The model under review builds one solid part; all positions refer to its coordinate system, in mm. Coordinates: 2 decimals unless noted, no trailing zeros. Loops run counter-clockwise (first coordinate to the right, second up) from the corner with the lowest first, then second, coordinate; pieces in that order, holes last. Notation, with made-up numbers: M -35,-4 L -9,-4 A37 cw -9,34 Z; hole C -6.5,87 d3. An arc over 180 degrees is marked long. Use CSV: the item, a comma, the result in double quotes. Start each with the question number.
1. Add section A-A, the plane z = 119.5. Write out the cut boundary in (x, y).
2. Clearance check with flat-ended pins moving along their axes: P1, Ø1, axis at x = 230, y = 199.5, coming from the +Z side; P2, Ø0.6, axis at x = 237.5, y = 199.5, coming from the -Z side; P3, Ø1, axis at x = 233, y = 181.5, coming from the +Z side; P4, Ø2, axis at x = 232.5, z = 51.5, coming from the +Y side. State where each tip first meets the part, or that it passes through.
3. For L1, parallel to X at y = 172.5, z = 68.5; L2, parallel to Z at x = 228.75, y = 191; L3, parallel to Y at x = 234.5, z = 143, list the stretches that pass through material, from the lowest coordinate up.
4. Add section B-B, the plane y = 180.5. Write out the cut boundary in (x, z).
5. Add section C-C, the plane z = 167. Write out the cut boundary in (x, y).
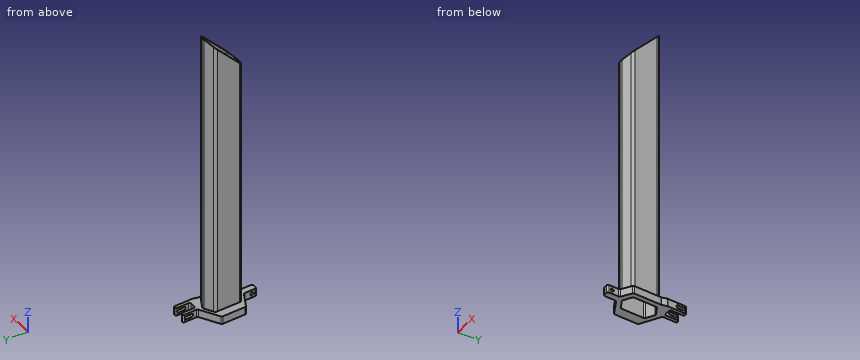
from build123d import *

# Parameters (mm, degrees)
BOSS_EXTRUDE1_DEPTH = 5
BOSS_EXTRUDE2_DEPTH = 180
SKETCH3_R           = 1
CUT_EXTRUDE1_DEPTH  = 180


with BuildPart() as part:
    # Sketch1 → Boss-Extrude1 (new body)
    with BuildSketch(Plane.XY):
        with BuildLine():
            Line((217.13080024, 186.236980413), (217.522895205, 171.902828405))
            ThreePointArc((217.522895205, 171.902828405), (217.676624689, 171.396825166), (218.066927795, 171.039984141))
            Line((218.066927795, 171.039984141), (227.253610039, 166.338288505))
            ThreePointArc((227.253610039, 166.338288505), (227.643913146, 165.981447481), (227.79764263, 165.475444242))
            Line((227.79764263, 165.475444242), (227.976831168, 158.924695096))
            ThreePointArc((227.976831168, 158.924695096), (228.279084932, 158.235329737), (228.97645726, 157.952038769))
            Line((228.97645726, 157.952038769), (230.8781853, 157.952038769))
            ThreePointArc((230.8781853, 157.952038769), (231.594894332, 158.254666441), (231.877811392, 158.979382441))
            Line((231.877811392, 158.979382441), (231.708538067, 165.167652598))
            ThreePointArc((231.708538067, 165.167652598), (231.820970232, 165.656392994), (232.156538916, 166.029088346))
            Line((232.156538916, 166.029088346), (237.939045309, 169.853338197))
            ThreePointArc((237.939045309, 169.853338197), (238.274613993, 170.226033549), (238.387046158, 170.714773945))
            Line((238.387046158, 170.714773945), (237.918224361, 187.853894574))
            ThreePointArc((237.918224361, 187.853894574), (237.922769134, 187.980299684), (237.94323412, 188.105119919))
            Line((237.94323412, 188.105119919), (238.683490474, 191.327652279))
            ThreePointArc((238.683490474, 191.327652279), (238.70395546, 191.452472514), (238.708500233, 191.578877624))
            Line((238.708500233, 191.578877624), (238.40594927, 202.639492732))
            ThreePointArc((238.40594927, 202.639492732), (238.093830671, 203.338326344), (237.37823169, 203.611754696))
            ThreePointArc((237.37823169, 203.611754696), (236.679398078, 203.299636096), (236.40594927, 202.584784932))
            Line((236.40594927, 202.584784932), (236.602823712, 195.38747707))
            ThreePointArc((236.602823712, 195.38747707), (236.329374904, 194.672625906), (235.630541293, 194.360507306))
            Line((235.630541293, 194.360507306), (232.531700408, 194.275741921))
            ThreePointArc((232.531700408, 194.275741921), (231.816849243, 194.549190729), (231.504730643, 195.248024341))
            Line((231.504730643, 195.248024341), (231.307856202, 202.445332202))
            ThreePointArc((231.307856202, 202.445332202), (230.995737602, 203.144165814), (230.280138621, 203.417594166))
            ThreePointArc((230.280138621, 203.417594166), (229.581305009, 203.105475566), (229.307856202, 202.390624402))
            Line((229.307856202, 202.390624402), (229.516006509, 194.781095054))
            ThreePointArc((229.516006509, 194.781095054), (229.392075465, 194.270886823), (229.026740392, 193.893790513))
            Line((229.026740392, 193.893790513), (217.620066357, 187.124284954))
            ThreePointArc((217.620066357, 187.124284954), (217.254731284, 186.747188644), (217.13080024, 186.236980413))
        make_face()
        with BuildLine():
            Line((228.516569513, 190.102489168), (223.742260028, 187.269085277))
            ThreePointArc((223.742260028, 187.269085277), (223.376924955, 186.891988967), (223.252993911, 186.381780736))
            Line((223.252993911, 186.381780736), (223.642537472, 172.14090257))
            ThreePointArc((223.642537472, 172.14090257), (223.796266956, 171.634899331), (224.186570063, 171.278058307))
            Line((224.186570063, 171.278058307), (229.107271966, 168.759668963))
            ThreePointArc((229.107271966, 168.759668963), (229.59020914, 168.650230807), (230.066441509, 168.785905991))
            Line((230.066441509, 168.785905991), (234.842112696, 171.569528957))
            ThreePointArc((234.842112696, 171.569528957), (235.212324771, 171.947173038), (235.338162748, 172.460823537))
            Line((235.338162748, 172.460823537), (234.948619186, 186.701701703))
            ThreePointArc((234.948619186, 186.701701703), (234.796981963, 187.204372068), (234.41157851, 187.560932751))
            Line((234.41157851, 187.560932751), (229.489514903, 190.12910302))
            ThreePointArc((229.489514903, 190.12910302), (228.999585816, 190.242154392), (228.516569513, 190.102489168))
        make_face(mode=Mode.SUBTRACT)
    extrude(amount=BOSS_EXTRUDE1_DEPTH)

    # Sketch2 → Boss-Extrude2 (add)
    with BuildSketch(Plane.XY.offset(5)):
        with BuildLine():
            Line((228.006209537, 190.962450037), (223.231900052, 188.129046145))
            ThreePointArc((223.231900052, 188.129046145), (222.501229906, 187.374853526), (222.253367819, 186.354437063))
            Line((222.253367819, 186.354437063), (222.642911381, 172.113558898))
            ThreePointArc((222.642911381, 172.113558898), (222.950370347, 171.10155242), (223.730976561, 170.387870371))
            Line((223.730976561, 170.387870371), (228.651678464, 167.869481027))
            ThreePointArc((228.651678464, 167.869481027), (229.617552813, 167.650604715), (230.57001755, 167.921955083))
            Line((230.57001755, 167.921955083), (235.345688737, 170.705578049))
            ThreePointArc((235.345688737, 170.705578049), (236.086112886, 171.460866211), (236.337788839, 172.48816721))
            Line((236.337788839, 172.48816721), (235.948245278, 186.729045376))
            ThreePointArc((235.948245278, 186.729045376), (235.644970831, 187.734386104), (234.874163925, 188.44750747))
            Line((234.874163925, 188.44750747), (229.952100319, 191.015677739))
            ThreePointArc((229.952100319, 191.015677739), (228.972242143, 191.241780484), (228.006209537, 190.962450037))
        make_face()
        with BuildLine():
            Line((223.252993911, 186.381780736), (223.642537472, 172.14090257))
            ThreePointArc((223.642537472, 172.14090257), (223.796266956, 171.634899331), (224.186570063, 171.278058307))
            Line((224.186570063, 171.278058307), (229.107271966, 168.759668963))
            ThreePointArc((229.107271966, 168.759668963), (229.59020914, 168.650230807), (230.066441509, 168.785905991))
            Line((230.066441509, 168.785905991), (234.842112696, 171.569528957))
            ThreePointArc((234.842112696, 171.569528957), (235.212324771, 171.947173038), (235.338162748, 172.460823537))
            Line((235.338162748, 172.460823537), (234.948619186, 186.701701703))
            ThreePointArc((234.948619186, 186.701701703), (234.796981963, 187.204372068), (234.41157851, 187.560932751))
            Line((234.41157851, 187.560932751), (229.489514903, 190.12910302))
            ThreePointArc((229.489514903, 190.12910302), (228.999585816, 190.242154392), (228.516569513, 190.102489168))
            Line((228.516569513, 190.102489168), (223.742260028, 187.269085277))
            ThreePointArc((223.742260028, 187.269085277), (223.376924955, 186.891988967), (223.252993911, 186.381780736))
        make_face(mode=Mode.SUBTRACT)
    extrude(amount=BOSS_EXTRUDE2_DEPTH)

    # Sketch3 → Cut-Extrude1 (cut)
    with BuildSketch(Plane(origin=(227.180903608, 6.214283783, 0), x_dir=(0, 0, 1), z_dir=(-0.999626092, -0.027343672, 0))):
        with Locations((2.5, 154.631921977)):
            Circle(SKETCH3_R)
        Polygon((185, 184.782926083), (185, 161.309331644), (160, 161.309331644), align=None)
        with BuildLine():
            Line((3.5, 195.044829999), (3.5, 191.544829999))
            ThreePointArc((3.5, 191.544829999), (2.5, 190.544829999), (1.5, 191.544829999))
            Line((1.5, 191.544829999), (1.5, 195.044829999))
            ThreePointArc((1.5, 195.044829999), (2.5, 196.044829999), (3.5, 195.044829999))
        make_face()
    extrude(amount=-CUT_EXTRUDE1_DEPTH, mode=Mode.SUBTRACT)


solid = part.part
Computed:
1,outline,"M 222.25,186.35 L 222.64,172.11 A2 ccw 223.73,170.39 L 228.65,167.87 A2 ccw 230.57,167.92 L 235.35,170.71 A2 ccw 236.34,172.49 L 235.95,186.73 A2 ccw 234.87,188.45 L 229.95,191.02 A2 ccw 228.01,190.96 L 223.23,188.13 A2 ccw Z; hole M 223.25,186.38 L 223.64,172.14 A1 ccw 224.19,171.28 L 229.11,168.76 A1 ccw 230.07,168.79 L 234.84,171.57 A1 ccw 235.34,172.46 L 234.95,186.7 A1 ccw 234.41,187.56 L 229.49,190.13 A1 ccw 228.52,190.1 L 223.74,187.27 A1 ccw Z"
2,P1,"stops at z = 5"
2,P2,"stops at z = 0"
2,P3,"passes through"
2,P4,"stops at y = 190.21"
3,L1,"x = 222.63 to 223.63, 235.34 to 236.34"
3,L2,"z = 0 to 184.88"
3,L3,"y = 170.21 to 171.37, 187.51 to 188.64"
4,outline,"M 217.29,0 L 223.41,0 L 223.41,173.86 L 222.41,173.89 L 222.41,5 L 217.29,5 Z; M 235.12,0 L 238.12,0 L 238.12,5 L 236.12,5 L 236.12,173.49 L 235.12,173.52 Z"
5,outline,"M 222.25,186.35 L 222.59,174.03 L 223.59,174.06 L 223.25,186.38 A1 cw 223.74,187.27 L 228.52,190.1 A1 cw 229.49,190.13 L 234.41,187.56 A1 cw 234.95,186.7 L 235.29,174.38 L 236.29,174.41 L 235.95,186.73 A2 ccw 234.87,188.45 L 229.95,191.02 A2 ccw 228.01,190.96 L 223.23,188.13 A2 ccw Z"
